```python
from build123d import *

# Parameters (mm, degrees)
SKETCH_1_W                   = 50
SKETCH_1_H                   = 45
EXTRUDE_1_DEPTH              = 6
HOLE_WIZARD_M3_1_D           = 3.4
HOLE_WIZARD_M3_1_CBORE_D     = 6.5
HOLE_WIZARD_M3_1_CBORE_DEPTH = 3.4
HOLE_WIZARD_M3_2_D           = 3.4
HOLE_WIZARD_M3_2_CBORE_D     = 6.5
HOLE_WIZARD_M3_2_CBORE_DEPTH = 3.4


with BuildPart() as part:
    # 草图1 → 凸台-拉伸1 (new body)
    with BuildSketch(Plane(origin=(0, 0, 0), x_dir=(1, 0, 0), z_dir=(0, 1, 0))):
        Rectangle(SKETCH_1_W, SKETCH_1_H)
    extrude(amount=EXTRUDE_1_DEPTH)

    # M3 六角凹头螺钉的柱形沉头孔1 (through all)
    with Locations(Plane(origin=(-20, 0, 17.5), x_dir=(0, 0, -1), z_dir=(0, -1, 0))):
        with Locations((0, 0), (0, 40), (35, 40), (35, 0)):
            CounterBoreHole(HOLE_WIZARD_M3_1_D / 2, HOLE_WIZARD_M3_1_CBORE_D / 2, HOLE_WIZARD_M3_1_CBORE_DEPTH)

    # M3 六角凹头螺钉的柱形沉头孔2 (through all)
    with Locations(Plane(origin=(-11, 6, -14), x_dir=(0, 0, 1), z_dir=(0, 1, 0))):
        with Locations((0, 0), (0, 20), (23.7, 10)):
            CounterBoreHole(HOLE_WIZARD_M3_2_D / 2, HOLE_WIZARD_M3_2_CBORE_D / 2, HOLE_WIZARD_M3_2_CBORE_DEPTH)


solid = part.part
```
Could you check a few things on this model? Use its own coordinates, in mm. A direction names the side the tool comes from. Round coordinates to 2 decimals unless told otherwise and drop trailing zeros. Loops run counter-clockwise (first coordinate to the right, second up) from the corner with the lowest first, then second, coordinate; pieces in that order, holes last.
Q1. Please list where these lines run through material, in increasing order: L1, parallel to X at y = 0.6, z = -14; L2, parallel to X at y = 5.15, z = -17.5; L3, parallel to Z at x = 20.5, y = 5.15.
Q2. Thinking about a two-plate mould opening in Z: for faces 1 (the cylindrical face through (-19.857, 1.676, 20.747)), 2 (the flat face through (0, 3, 22.5)), 3 (the flat face through (0, 3, -22.5)), 4 (the flat face through (25, 3, 0)), which applies, pulls with the +Z half, pulls with the -Z half, needs draft (parallel to the pull), parting line crosses it, or undercut?
Q3. I want a section at C-C (z = 9.7). Write out the boundary of the cut face in (x, y).
Q4. I want a section at D-D (x = 20). Write out the boundary of the cut face in (y, z), and give its area (3 significant figures).
Q5. I want a section at B-B (y = 4.3). Write out the boundary of the cut face in (x, z), and give its area (3 significant figures).
Q6. On a 3-axis mill with a long thin cutter (end or side, diameter ignored), from which of +Z, -Z, +X, -X, +Y, -Y can I reach the whole of each face in a straight line? I mean faces 5 (the cylindrical face through (-2.03, 1.28, 11.05)), 6 (the cylindrical face through (20.143, 1.676, 20.747)), 7 (the flat face through (7.6, 2.6, -12.6)). Say none if no direction works.
Q7. I want a section at A-A (x = -1). Write out the boundary of the cut face in (y, z).
Q8. For P1, Ø4.5, axis at x = 20, z = 17.5, coming from the +Y side; P2, Ø2, axis at x = 7.5, z = -15, coming from the +Y side; P3, Ø3, axis at x = -11, z = -14, coming from the +Y side, each with a flat end and sliding along its axis, tell me the tip position at first contact or that it passes through.
Answer below:
1. L1: x = -25 to -12.7, -9.3 to 7.3, 10.7 to 25
1. L2: x = -25 to -21.7, -18.3 to 18.3, 21.7 to 25
1. L3: z = -22.5 to -19.12, -15.88 to 15.88, 19.12 to 22.5
2. face 1: undercut
2. face 2: pulls with the +Z half
2. face 3: pulls with the -Z half
2. face 4: needs draft
3. outline: (-25, 0) - (-2.7, 0) - (-2.7, 2.6) - (-4.25, 2.6) - (-4.25, 6) - (-25, 6) - close; (0.7, 0) - (25, 0) - (25, 6) - (2.25, 6) - (2.25, 2.6) - (0.7, 2.6) - close
4. outline: (0, -22.5) - (6, -22.5) - (6, -19.2) - (3.4, -19.2) - (3.4, -20.75) - (0, -20.75) - close; (0, -14.25) - (3.4, -14.25) - (3.4, -15.8) - (6, -15.8) - (6, 15.8) - (3.4, 15.8) - (3.4, 14.25) - (0, 14.25) - close; (0, 20.75) - (3.4, 20.75) - (3.4, 19.2) - (6, 19.2) - (6, 22.5) - (0, 22.5) - close
4. area: 208 mm2
5. outline: (-25, -22.5) - (25, -22.5) - (25, 22.5) - (-25, 22.5) - close; hole circle Ø3.4 at (-20, -17.5); hole circle Ø3.4 at (-20, 17.5); hole circle Ø6.5 at (-11, -14); hole circle Ø6.5 at (-1, 9.7); hole circle Ø6.5 at (9, -14); hole circle Ø3.4 at (20, -17.5); hole circle Ø3.4 at (20, 17.5)
5. area: 2,110 mm2
6. face 5: +Y, -Y
6. face 6: -Y
6. face 7: +Y
7. outline: (0, -22.5) - (6, -22.5) - (6, 6.45) - (2.6, 6.45) - (2.6, 8) - (0, 8) - close; (0, 11.4) - (2.6, 11.4) - (2.6, 12.95) - (6, 12.95) - (6, 22.5) - (0, 22.5) - close
8. P1: stops at y = 6
8. P2: stops at y = 2.6
8. P3: passes through
